CAD build for the part. Positions are in the model's coordinates, mm. A direction names the side the tool comes from. Give positions to 0.01 mm unless a question says otherwise; leave off trailing zeros. Loops run counter-clockwise (first coordinate to the right, second up) from the corner with the lowest first, then second, coordinate; pieces in that order, holes last. Notation, with made-up numbers: M 5.25,60.25 L 25.25,60.25 A23 ccw 25.25,71.25 Z; hole C 26.25,31.25 d5. An arc over 180 degrees is marked long. One line per question, with ' | ' between items.
```python
from build123d import *

# Parameters (mm, degrees)
F0_R     = 5
F1_DEPTH = 60
F3_W     = 226.6252040863
F3_H     = 197.2780163714
F3_H_2   = 59.4672214857
F4_DEPTH = 35
F5_R     = 75
F6_SIZE  = 12


# Not quite as in the source:
# - a feature names something its author has since deleted; it is built from what else it names


with BuildPart() as f1:
    # F0 (on Right) → F1 (new body, symmetric)
    with BuildSketch(Plane.YZ):
        Polygon((-87.5, -90), (-87.5, -170), (87.5, -170), (87.5, -90), (50, 130), (-50, 130), align=None)
        with Locations((0, -90)):
            Circle(F0_R, mode=Mode.SUBTRACT)
    extrude(amount=F1_DEPTH, both=True)

    # F3 (on face) → F4 (cut, symmetric)
    with BuildSketch(Plane.YZ):
        with Locations((-5.2212774754, -37.3711218749)):
            Rectangle(F3_W, F3_H)
        with Locations((-5.2212774754, -165.7437408035)):
            Rectangle(F3_W, F3_H_2)
    extrude(amount=F4_DEPTH, both=True, mode=Mode.SUBTRACT)

    # F5
    f5_edges = [f1.edges().sort_by_distance(p)[0] for p in [
        (-47.5, 87.5, -170),
        (47.5, 87.5, -170),
        (47.5, -87.5, -170),
        (-47.5, -87.5, -170),
    ]]
    fillet(f5_edges, radius=F5_R)

    # F6
    f6_edges = [f1.edges().sort_by_distance(p)[0] for p in [
        (60, 68.75, 20),
        (-60, 68.75, 20),
        (60, -65.533009, -148.033009),
        (60, -68.75, 20),
        (-60, -65.533009, -148.033009),
        (-60, -68.75, 20),
    ]]
    chamfer(f6_edges, length=F6_SIZE)


solid = f1.part
```
Item 1: Mould opens along Z. For faces 3 (the cylindrical face through (-41.41, -66.11, -147.45)), 4 (the flat face through (53.9, -81.6, -92.5)), 5 (the cylindrical face through (-47.68, -1.08, -94.88)) say: pulls with the +Z half, pulls with the -Z half, needs draft (parallel to the pull), parting line crosses it, or undercut.
Conclusion:
face 3: pulls with the -Z half | face 4: needs draft | face 5: undercut
Item 2: 3-axis set-ups, long thin cutter, end or side, ignore diameter. For faces 1 (the flat face through (54, 0, -164)), 2 (the flat face through (-35, -1, -53)): which of +Z, -Z, +X, -X, +Y, -Y reach the whole face in a straight line?
Conclusion:
face 1: -Z, +X, +Y, -Y | face 2: -Z, +Y, -Y
Item 3: Saw through at B-B on z = 109. Give the cut face in (x, y).
Conclusion:
outline: M -60,-41.41 L -48,-53.58 L 48,-53.58 L 60,-41.41 L 60,41.41 L 48,53.58 L -48,53.58 L -60,41.41 Z
Item 4: Saw through at A-A on y = 0. Give the cut face in (x, z), and give its area (3 significant figures).
Conclusion:
outline: M -60,-158 L -48,-170 L -35,-170 L -35,-95 L -60,-95 Z; M -60,-85 L -35,-85 L -35,61.27 L 35,61.27 L 35,-85 L 60,-85 L 60,130 L -60,130 Z; M 35,-170 L 48,-170 L 60,-158 L 60,-95 L 35,-95 Z | area: 19,200 mm²
Item 5: Saw through at C-C on x = -19.5. Give the cut face in (y, z).
Conclusion:
outline: M -61.72,61.27 L 61.72,61.27 L 50,130 L -50,130 Z
Item 6: Drop flat-ended pins along their axis: P1, Ø13, axis at y = 0, z = -90, coming from the +X side; P2, Ø8, axis at y = 63.5, z = 51, coming from the +X side; P3, Ø2, axis at x = -48, z = -75.5, coming from the +Y side. Give the stop position or say it passes through.
Conclusion:
P1: x = 60 | P2: x = 51.97 | P3: y = 85.2
Item 7: Drill centre lines: line 1 along X through (y, z) = (55, -103); line 2 along Y through (x, z) = (42.75, -90); line 3 along Z through (x, y) = (48, 0). Where is each one in solid material? Low to high. Write a range as [from, to].
Conclusion:
line 1: [-60, -35], [35, 60] | line 2: [-87.5, -5], [5, 87.5] | line 3: [-170, -95], [-85, 130]
